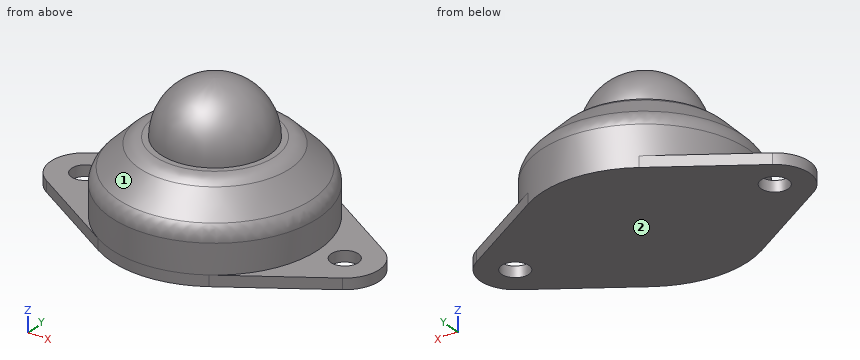
from build123d import *

# Parameters (mm, degrees)
F0_R     = 2
F1_DEPTH = 1.5875
F2_R     = 15.24
F3_DEPTH = 10.7315
F4_R     = 8.001
F5_DEPTH = 8.001
F6_R     = 8.00099
F7_SIZE  = 5.08
F8_R     = 3.175


# Not quite as in the source:
# - a fillet or chamfer is up to 0.001 mm smaller than in the source, because OpenCascade refuses the exact size


with BuildPart() as f1:
    # F0 (on Top) → F1 (new body)
    with BuildSketch(Plane.XY):
        with BuildLine():
            Line((10.922, 12.8915947811), (-2.7093333333, 4.2971982604))
            ThreePointArc((-2.7093333333, 4.2971982604), (-5.08, 0), (-2.7093333333, -4.2971982604))
            Line((-2.7093333333, -4.2971982604), (10.922, -12.8915947811))
            ThreePointArc((10.922, -12.8915947811), (19.05, -15.24), (27.178, -12.8915947811))
            Line((27.178, -12.8915947811), (40.8093333333, -4.2971982604))
            ThreePointArc((40.8093333333, -4.2971982604), (43.18, 0), (40.8093333333, 4.2971982604))
            Line((40.8093333333, 4.2971982604), (27.178, 12.8915947811))
            ThreePointArc((27.178, 12.8915947811), (19.05, 15.24), (10.922, 12.8915947811))
        make_face()
        Circle(F0_R, mode=Mode.SUBTRACT)
        with Locations((38.1, 0)):
            Circle(F0_R, mode=Mode.SUBTRACT)
    extrude(amount=F1_DEPTH)

    # F2 (on face) → F3 (join)
    with BuildSketch(Plane.XY.offset(1.5875)):
        with Locations((19.05, 0)):
            Circle(F2_R)
    extrude(amount=F3_DEPTH)

    # F4 (on face) → F5 (join)
    with BuildSketch(Plane.XY.offset(12.319)):
        with Locations((19.05, 0)):
            Circle(F4_R)
    extrude(amount=F5_DEPTH)

    # F6 (radius 8.001 in the source; OpenCascade refuses exactly that, so slightly less here)
    f6_edges = [f1.edges().sort_by_distance(p)[0] for p in [
        (11.049, 0, 20.32),
    ]]
    fillet(f6_edges, radius=F6_R)

    # F7
    f7_edges = [f1.edges().sort_by_distance(p)[0] for p in [
        (3.81, 0, 12.319),
    ]]
    chamfer(f7_edges, length=F7_SIZE)

    # F8
    f8_edges = [f1.edges().sort_by_distance(p)[0] for p in [
        (3.81, 0, 7.239),
        (8.89, 0, 12.319),
    ]]
    fillet(f8_edges, radius=F8_R)


solid = f1.part
Geometry: final body of the model. Coordinates: model frame, mm. Face numbers are marked on the shaded views. Give positions to 0.01 mm unless a question says otherwise; leave off trailing zeros. Loops run counter-clockwise (first coordinate to the right, second up) from the corner with the lowest first, then second, coordinate; pieces in that order, holes last. Notation, with made-up numbers: (29, 24) - (38, 24) arc R18 cw to (38, 32) - close; hole circle Ø9 at (-28.75, 67). An arc over 180 degrees is marked (long way). Answer as CSV lines item,"result". Start each with the question number.
1. Pin query (flat end, axial travel): P1, Ø6, axis at x = 17, z = 17.5, coming from the +Y side; P2, Ø4.5, axis at x = 0, y = 0, coming from the +Z side; P3, Ø8, axis at x = 6.5, y = -5, coming from the +Z side; P4, Ø2.5, axis at x = 38.1, y = 0, coming from the -Z side. Return the tip coordinate at first contact, or that it passes through.
2. Section A-A, the plane x = 0. Return loops of the section in (y, z).
3. Draft query along Y for the marked faces 1 and 2. Return one class per face: released by +Y, released by -Y, zero draft, split by the parting line, or undercut.
4. Ray query, L1, parallel to Y at x = 38.1, z = 0.5; L2, parallel to Z at x = -0.5, y = 3.5; L3, parallel to Z at x = 8.5, y = -2.5. Return the intervals inside material, ascending.
Answers:
1,P1,"stops at y = 7.58"
1,P2,"stops at z = 1.59"
1,P3,"stops at z = 12.25"
1,P4,"passes through"
2,outline,"(-6.01, 0) - (-2, 0) - (-2, 1.59) - (-6.01, 1.59) - close; (2, 0) - (6.01, 0) - (6.01, 1.59) - (2, 1.59) - close"
3,face 1,"split by the parting line"
3,face 2,"zero draft"
4,L1,"y = -6.01 to -2, 2 to 6.01"
4,L2,"z = 0 to 1.59"
4,L3,"z = 0 to 11.61"
